Build history of the part. All positions in model axes, mm. A direction names the side the tool comes from. Give positions to 0.01 mm unless a question says otherwise; leave off trailing zeros. Loops run counter-clockwise (first coordinate to the right, second up) from the corner with the lowest first, then second, coordinate; pieces in that order, holes last. Notation, with made-up numbers: (-33, -26.5) -> (12, -26.5) arc R8 ccw to (12, -12.5) -> close; hole circle Ø3 at (59.25, -38). An arc over 180 degrees is marked (long way). One line per question, with ' | ' between items. Start each with the question number.
(1) Slice it at D-D, the plane y = 2.5. Write the cut outline in (x, z).
(2) 3-axis set-ups, long thin cutter, end or side, ignore diameter. For faces 5 (the face through (-8.444, 3, 2)), 6 (the face through (-2, 4, 0)): which of +Z, -Z, +X, -X, +Y, -Y reach the whole face in a straight line?
(3) Drill centre lines: L1, parallel to Z at x = -1.25, y = 1; L2, parallel to X at y = 3.75, z = -0.75; L3, parallel to Y at x = -3.75, z = 0. Where is each one in solid material? Low to high. Write a range as from..to.
(4) Slice it at B-B, the plane z = 7. Write the cut outline in (x, y).
(5) Slice it at C-C, the plane x = 4. Write the cut outline in (y, z), then the cut area to 3 significant figures.
(6) Flat gauge pins, fed straight in: pin 1 Ø9 at (x, z) = (2, 3) entering from -Y; pin 2 Ø2 at (x, z) = (5, -1.5) entering from -Y. Where does each tip first touch, or does it go through?
(7) Mould opens along X. For faces 1 (the face through (-0.119, 2, 1)), 2 (the face through (-7.874, 3.042, 10.314)), 3 (the face through (2, 0, 3)), 4 (the face through (2, 2, 2.59)) say: pulls with the +X half, pulls with the -X half, needs draft (parallel to the pull), parting line crosses it, or undercut.
(8) Slice it at A-A, the plane y = 1.25. Write the cut outline in (x, z), then the cut area to 3 significant figures.
```python
from build123d import *

# Parameters (mm, degrees)
SKETCH1_W           = 18
SKETCH1_H           = 18
BOSS_EXTRUDE1_DEPTH = 6
SKETCH2_W           = 14
SKETCH2_H           = 14
CUT_EXTRUDE1_DEPTH  = 4
CUT_EXTRUDE1_DRAFT  = -20
SKETCH3_R           = 3
BOSS_EXTRUDE2_DEPTH = 4
FILLET1_R           = 2


with BuildPart() as part:
    # Sketch1 → Boss-Extrude1 (new body)
    with BuildSketch(Plane(origin=(0, 0, 0), x_dir=(1, 0, 0), z_dir=(0, 1, 0))):
        with Locations((0.556064073, -1.915331808)):
            Rectangle(SKETCH1_W, SKETCH1_H)
    extrude(amount=BOSS_EXTRUDE1_DEPTH)


with BuildPart() as cut_extrude1_tool:
    # Sketch2 → Cut-Extrude1 (with draft: the straight prism first)
    with BuildSketch(Plane.XZ):
        with Locations((0.556064073, 1.915331808)):
            Rectangle(SKETCH2_W, SKETCH2_H)
    extrude(amount=-CUT_EXTRUDE1_DEPTH)
    # Cut-Extrude1: the draft: its side faces are tilted about the plane it starts from
    cut_extrude1_sides = [cut_extrude1_tool.faces().sort_by_distance(p)[0] for p in [
        (-6.443935927, 2, 1.915331808),
        (0.556064073, 2, -5.084668192),
        (7.556064073, 2, 1.915331808),
        (0.556064073, 2, 8.915331808),
    ]]
    draft(cut_extrude1_sides, Plane.XZ, CUT_EXTRUDE1_DRAFT)


with BuildPart() as part_1:
    add(part.part)

    # Cut-Extrude1: cut by cut_extrude1_tool
    add(cut_extrude1_tool.part, mode=Mode.SUBTRACT)

    # Sketch3 → Boss-Extrude2 (add)
    with BuildSketch(Plane.XZ.offset(-4)):
        with Locations(Location((0.556064073, 1.915331808, 0), (0, 0, 270))):
            Circle(SKETCH3_R)
        Polygon((-0.118935927, 1.240331808), (-1.468935927, 1.240331808), (-1.468935927, 2.590331808), (-0.118935927, 2.590331808), (-0.118935927, 3.940331808), (1.231064073, 3.940331808), (1.231064073, 2.590331808), (2.581064073, 2.590331808), (2.581064073, 1.240331808), (1.231064073, 1.240331808), (1.231064073, -0.109668192), (-0.118935927, -0.109668192), align=None, mode=Mode.SUBTRACT)
    extrude(amount=BOSS_EXTRUDE2_DEPTH)

    # Fillet1
    fillet1_edges = [part_1.edges().sort_by_distance(p)[0] for p in [
        (-8.443935927, 3, -7.084668192),
        (9.556064073, 3, -7.084668192),
        (9.556064073, 3, 10.915331808),
        (-8.443935927, 3, 10.915331808),
    ]]
    fillet(fillet1_edges, radius=FILLET1_R)


solid = part_1.part
```
Final values:
1) outline: (-8.44, -5.08) arc R2 ccw to (-6.44, -7.08) -> (7.56, -7.08) arc R2 ccw to (9.56, -5.08) -> (9.56, 8.92) arc R2 ccw to (7.56, 10.92) -> (-6.44, 10.92) arc R2 ccw to (-8.44, 8.92) -> close; circle Ø6 at (0.56, 1.92); hole (-5.53, -4.17) -> (6.65, -4.17) -> (6.65, 8.01) -> (-5.53, 8.01) -> close; hole (-1.47, 1.24) -> (-0.12, 1.24) -> (-0.12, -0.11) -> (1.23, -0.11) -> (1.23, 1.24) -> (2.58, 1.24) -> (2.58, 2.59) -> (1.23, 2.59) -> (1.23, 3.94) -> (-0.12, 3.94) -> (-0.12, 2.59) -> (-1.47, 2.59) -> close
2) face 5: +Z, -Z, -X, +Y, -Y | face 6: -Y
3) L1: -7.08..-4.72, -0.48..1.24, 2.59..4.31, 8.55..10.92 | L2: -8.44..-5.08, -0.82..1.93, 6.19..9.56 | L3: 4..6
4) outline: (-8.44, 0) -> (-6.44, 0) -> (-4.99, 4) -> (6.1, 4) -> (7.56, 0) -> (9.56, 0) -> (9.56, 6) -> (-8.44, 6) -> close
5) outline: (0, -7.08) -> (6, -7.08) -> (6, 10.92) -> (0, 10.92) -> (0, 8.92) -> (4, 7.46) -> (4, -3.63) -> (0, -5.08) -> close | area: 57.8 mm2
6) pin 1: y = 0 | pin 2: y = 4
7) face 1: undercut | face 2: pulls with the -X half | face 3: needs draft | face 4: undercut
8) outline: (-8.44, -5.08) arc R2 ccw to (-6.44, -7.08) -> (7.56, -7.08) arc R2 ccw to (9.56, -5.08) -> (9.56, 8.92) arc R2 ccw to (7.56, 10.92) -> (-6.44, 10.92) arc R2 ccw to (-8.44, 8.92) -> close; circle Ø6 at (0.56, 1.92); hole (-5.99, -4.63) -> (7.1, -4.63) -> (7.1, 8.46) -> (-5.99, 8.46) -> close; hole (-1.47, 1.24) -> (-0.12, 1.24) -> (-0.12, -0.11) -> (1.23, -0.11) -> (1.23, 1.24) -> (2.58, 1.24) -> (2.58, 2.59) -> (1.23, 2.59) -> (1.23, 3.94) -> (-0.12, 3.94) -> (-0.12, 2.59) -> (-1.47, 2.59) -> close | area: 168 mm2
